Drawing for the job (mm, zero at the part's lowest x, y, z). Give positions to 0.01 mm unless a question says otherwise; leave off trailing zeros. Order: outer loops, then holes, each group sorted by start corner. A loop starts at its lowest first (then second) coordinate and runs counter-clockwise, first axis right, second up. Notation, with made-up numbers: (48.5, 36.5) - (104.5, 36.5) arc R18 ccw to (104.5, 66.5) - close; hole circle Ø6 at (78.25, -19.75). An arc over 180 degrees is marked (long way). One line per item, written item: value.
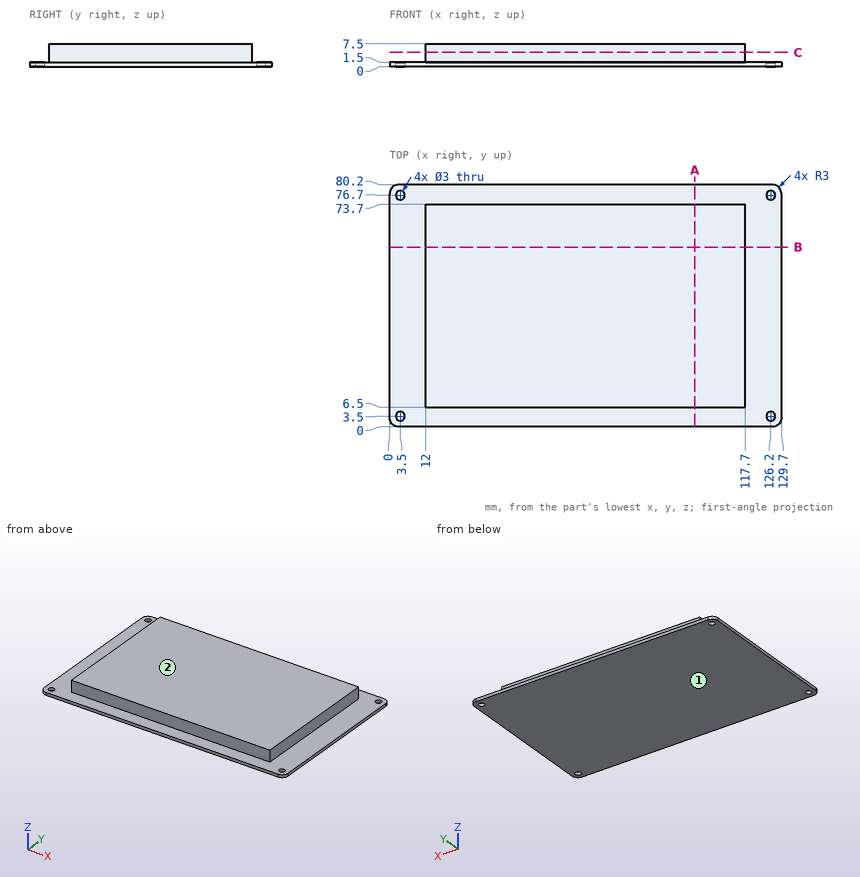
(1) Pull direction Z, two halves, no side cores. Call the marked faces 1 and 2: +Z half, -Z half, draft (parallel to the pull), parting line (faces both ways), or undercut.
Completed:
face 1: -Z half
face 2: +Z half
(2) Drill centre lines: line 1 (Y direction, x = 3.5, z = 0.9); line 2 (Y direction, x = 42, z = 2.75); line 3 (Z direction, x = 122, y = 30.5). Where is each one in solid material? Low to high.
Completed:
line 1: 0 to 2, 5 to 75.2, 78.2 to 80.2
line 2: 6.5 to 73.7
line 3: 0 to 1.5
(3) Slice it at C-C, the plane z = 4.75. Give the cut face in (x, y).
Completed:
outline: (12, 6.5) - (117.7, 6.5) - (117.7, 73.7) - (12, 73.7) - close
(4) Slice it at B-B, the plane y = 59.5. Give the cut face in (x, z).
Completed:
outline: (0, 0) - (129.7, 0) - (129.7, 1.5) - (117.7, 1.5) - (117.7, 7.5) - (12, 7.5) - (12, 1.5) - (0, 1.5) - close
(5) Slice it at A-A, the plane x = 101. Give the cut face in (y, z), and give its area (4 significant figures).
Completed:
outline: (0, 0) - (80.2, 0) - (80.2, 1.5) - (73.7, 1.5) - (73.7, 7.5) - (6.5, 7.5) - (6.5, 1.5) - (0, 1.5) - close
area: 523.5 mm²
(6) Pin check, flat tips, straight feed: P1, Ø1.8, axis at y = 29, z = 5, coming from the -X side; P2, Ø2.5, axis at x = 126.2, y = 76.7, coming from the -Z side; P3, Ø4, axis at x = 13.5, z = 5.5, coming from the -Y side; P4, Ø1.8, axis at y = 38, z = 3, coming from the +X side. Stop position of each tip, or through.
Completed:
P1: x = 12
P2: through
P3: y = 6.5
P4: x = 117.7
